The figure shows three views and two pictorial views of one solid part (mm, origin at its lowest corner). Answer the questions. A direction names the side the tool comes from. Coordinates: 2 decimals unless noted, no trailing zeros. Loops run counter-clockwise (first coordinate to the right, second up) from the corner with the lowest first, then second, coordinate; pieces in that order, holes last. Notation, with made-up numbers: (72.5, 1.25) -> (99.5, 1.25) arc R33 cw to (99.5, 31.25) -> close; hole circle Ø9 at (84, 57). An arc over 180 degrees is marked (long way). Answer in a Markdown table with one row per item.
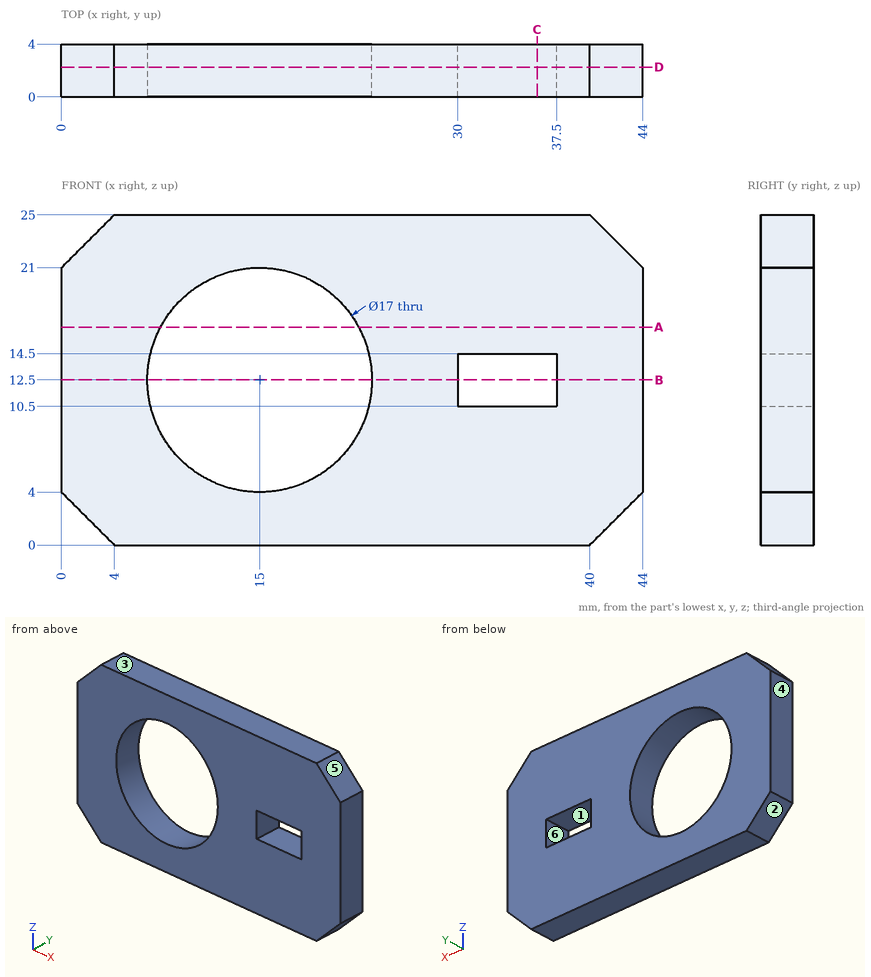
Item 1: A cutting plane is placed at D-D, the plane y = 2.25. Determine the outline of the cut face in (x, z), plus the area to 3 significant figures.
Findings below:
| item | result |
|---|---|
| outline | (0, 4) -> (4, 0) -> (40, 0) -> (44, 4) -> (44, 21) -> (40, 25) -> (4, 25) -> (0, 21) -> close; hole circle Ø17 at (15, 12.5); hole (30, 10.5) -> (37.5, 10.5) -> (37.5, 14.5) -> (30, 14.5) -> close |
| area | 811 mm2 |
Item 2: A cutting plane is placed at C-C, the plane x = 36. Determine the outline of the cut face in (y, z), plus the area to 3 significant figures.
Findings below:
| item | result |
|---|---|
| outline | (0, 0) -> (4, 0) -> (4, 10.5) -> (0, 10.5) -> close; (0, 14.5) -> (4, 14.5) -> (4, 25) -> (0, 25) -> close |
| area | 84.0 mm2 |
Item 3: Determine the mould class of the marked faces 3, 4, 5 and 6 for opening direction X: +X half, -X half, draft (parallel to the pull), parting line (faces both ways), or undercut.
Findings below:
| item | result |
|---|---|
| face 3 | draft |
| face 4 | -X half |
| face 5 | +X half |
| face 6 | undercut |
Item 4: A tool of negligible diameter and unlimited length cuts with its end or side. For the marked faces 1 and 2, from which of +Z, -Z, +X, -X, +Y, -Y can it reach the whole face along a straight path? Write none if from no direction.
Findings below:
| item | result |
|---|---|
| face 1 | +Y, -Y |
| face 2 | -Z, -X, +Y, -Y |
Item 5: A cutting plane is placed at A-A, the plane z = 16.5. Determine the outline of the cut face in (x, y).
Findings below:
| item | result |
|---|---|
| outline | (0, 0) -> (7.5, 0) -> (7.5, 4) -> (0, 4) -> close; (22.5, 0) -> (44, 0) -> (44, 4) -> (22.5, 4) -> close |
Item 6: A cutting plane is placed at B-B, the plane z = 12.5. Determine the outline of the cut face in (x, y), plus the area to 3 significant figures.
Findings below:
| item | result |
|---|---|
| outline | (0, 0) -> (6.5, 0) -> (6.5, 4) -> (0, 4) -> close; (23.5, 0) -> (30, 0) -> (30, 4) -> (23.5, 4) -> close; (37.5, 0) -> (44, 0) -> (44, 4) -> (37.5, 4) -> close |
| area | 78.0 mm2 |
Item 7: Find the intervals of material crossed by probe 1 along X at (y, z) = (1.4, 12.5); probe 2 along Z at (x, y) = (15, 2.1); probe 3 along Z at (x, y) = (33, 2.4), in increasing order.
Findings below:
| item | result |
|---|---|
| probe 1 | x = 0 to 6.5, 23.5 to 30, 37.5 to 44 |
| probe 2 | z = 0 to 4, 21 to 25 |
| probe 3 | z = 0 to 10.5, 14.5 to 25 |
